Model file for the job. Use its own axes, mm. A direction names the side the tool comes from. Round coordinates to 2 decimals unless told otherwise and drop trailing zeros. Loops run counter-clockwise (first coordinate to the right, second up) from the corner with the lowest first, then second, coordinate; pieces in that order, holes last. Notation, with made-up numbers: (-0.5, -21) - (57.5, -21) arc R35 cw to (57.5, 12) - close; hole circle Ø1 at (24, -1). An arc over 180 degrees is marked (long way). Use one line per item in the form item = value.
from build123d import *

# Parameters (mm, degrees)
SKETCH1_R                   = 12.7
BOSS_EXTRUDE1_DEPTH         = 101.6
F_1_2_20_TAPPED_HOLE1_D     = 11.50874
F_1_2_20_TAPPED_HOLE1_DEPTH = 38.1
F_1_2_20_TAPPED_HOLE1_TIP   = 3.45757432
F_1_2_20_TAPPED_HOLE2_D     = 11.50874
F_1_2_20_TAPPED_HOLE2_DEPTH = 38.1
F_1_2_20_TAPPED_HOLE2_TIP   = 3.45757432
CHAMFER1_SIZE               = 2.54


with BuildPart() as part:
    # Sketch1 → Boss-Extrude1 (new body)
    with BuildSketch(Plane(origin=(0, 0, 0), x_dir=(1, 0, 0), z_dir=(0, 1, 0))):
        with Locations(Location((0, 0, 0), (0, 0, 270))):
            Circle(SKETCH1_R)
    extrude(amount=BOSS_EXTRUDE1_DEPTH)

    # 1/2-20 Tapped Hole1
    with Locations(Plane.ZX.offset(101.6)):
        with Locations((0, 0)):
            Hole(F_1_2_20_TAPPED_HOLE1_D / 2, depth=F_1_2_20_TAPPED_HOLE1_DEPTH)
            with Locations((0, 0, -(F_1_2_20_TAPPED_HOLE1_DEPTH + F_1_2_20_TAPPED_HOLE1_TIP / 2))):  # 118° drill point
                Cone(0, F_1_2_20_TAPPED_HOLE1_D / 2, F_1_2_20_TAPPED_HOLE1_TIP, mode=Mode.SUBTRACT)

    # 1/2-20 Tapped Hole2
    with Locations(Plane(origin=(0, 0, 0), x_dir=(0, 0, -1), z_dir=(0, -1, 0))):
        with Locations((0, 0)):
            Hole(F_1_2_20_TAPPED_HOLE2_D / 2, depth=F_1_2_20_TAPPED_HOLE2_DEPTH)
            with Locations((0, 0, -(F_1_2_20_TAPPED_HOLE2_DEPTH + F_1_2_20_TAPPED_HOLE2_TIP / 2))):  # 118° drill point
                Cone(0, F_1_2_20_TAPPED_HOLE2_D / 2, F_1_2_20_TAPPED_HOLE2_TIP, mode=Mode.SUBTRACT)

    # Chamfer1
    chamfer1_edges = [part.edges().sort_by_distance(p)[0] for p in [
        (0, 0, -12.7),
        (0, 101.6, -12.7),
    ]]
    chamfer(chamfer1_edges, length=CHAMFER1_SIZE)


solid = part.part
1. Pull direction X, two halves, no side cores. Call faces 4 (the conical face through (-0.976, 40.957, 0.217)), 5 (the flat face through (-4.4, 0, 4.4)), 6 (the conical face through (3.089, 0.123, 9.808)): +X half, -X half, draft (parallel to the pull), parting line (faces both ways), or undercut.
Geometry check:
face_4 = undercut
face_5 = draft
face_6 = parting line
2. Flat gauge pins, fed straight in: pin 1 (12 mm diameter, centred on y = 45, z = -6, fed in from -X); pin 2 (2 mm diameter, centred on y = 33, z = -8.5, fed in from +X); pin 3 (10 mm diameter, centred on y = 63.5, z = 9.5, fed in from -X); pin 4 (4 mm diameter, centred on y = 75.5, z = 6.5, fed in from +X). Where does each tip first touch, or does it go through?
Geometry check:
pin_1 = -12.7
pin_2 = 10.25
pin_3 = -11.88
pin_4 = 11.88
3. Cut at B-B, the plane y = 50. Give the cut face in (x, z), plus the area to 3 significant figures.
Geometry check:
outline = circle Ø25.4 at (0, 0)
area = 507 mm^2
4. Tool access for faces 1 (the cylindrical face through (5.705, 82.283, 0.749)), 2 (the cylindrical face through (-7.7, 50.1, -10.1)), 3 (the cylindrical face through (5.705, 19.317, -0.749)): list every direction of +Z, -Z, +X, -X, +Y, -Y with a clear straight run to the whole face (end or side of a thin tool).
Geometry check:
face_1 = +Y
face_2 = +Y, -Y
face_3 = -Y
5. Wall check: probe 1 along X at (y, z) = (13.5, 0); probe 2 along X at (y, z) = (56, -0.5). Give the ranges that are in metal, low to high.
Geometry check:
probe_1 = -12.7 to -5.75, 5.75 to 12.7
probe_2 = -12.69 to 12.69
6. Cut at A-A, the plane y = 94. Give the cut face in (x, z), plus the area to 3 significant figures.
Geometry check:
outline = circle Ø25.4 at (0, 0); hole circle Ø11.51 at (0, 0)
area = 403 mm^2
